Can you work these out from the drawing? Everything is in mm from the part's minimum corner. A direction names the side the tool comes from. Coordinates: 2 decimals unless noted, no trailing zeros. Loops run counter-clockwise (first coordinate to the right, second up) from the corner with the lowest first, then second, coordinate; pieces in that order, holes last. Notation, with made-up numbers: M -16,-13.75 L 1,-13.75 A20 ccw 1,0.25 Z; hole C 3,69 d5. An arc over 180 degrees is marked long. Write each question's results on one line, items separated by ' | '.
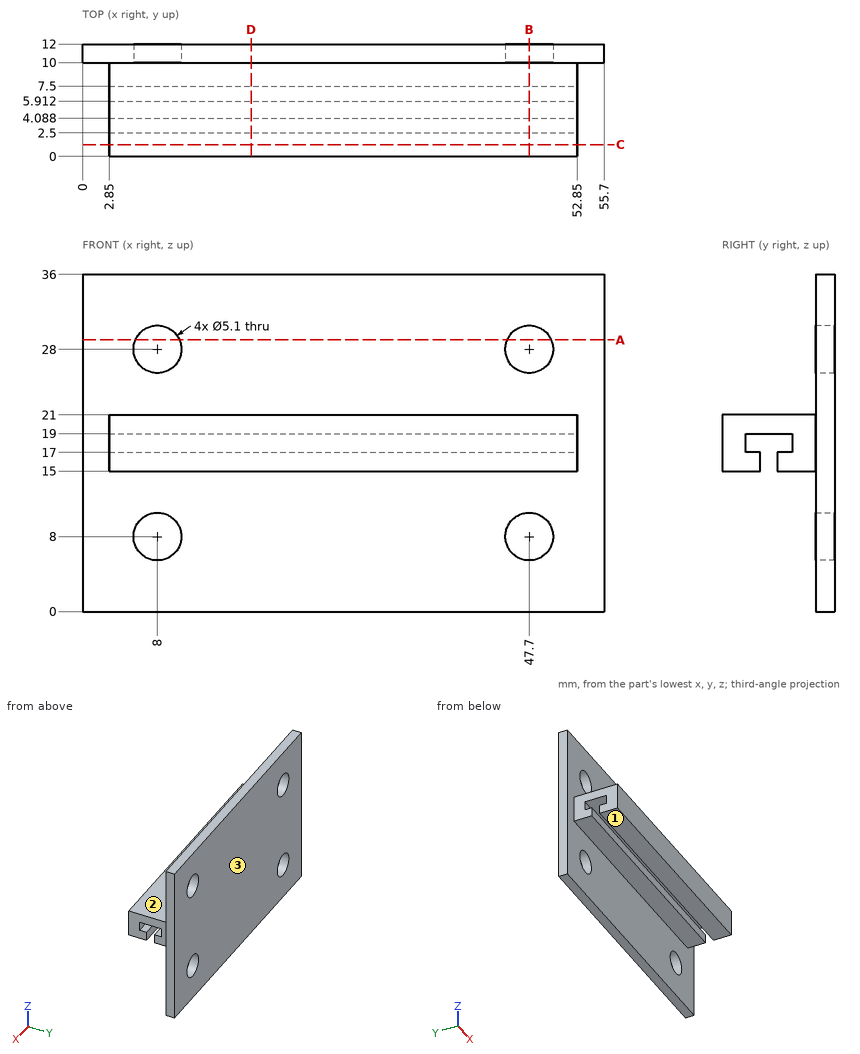
(1) Imagine slicing it at A-A, the plane z = 29. List the corners of the cut face in (x, y) for me (1 decimal).
Reported:
outline: M 0,10 L 5.7,10 L 5.7,12 L 0,12 Z; M 10.3,10 L 45.4,10 L 45.4,12 L 10.3,12 Z; M 50,10 L 55.7,10 L 55.7,12 L 50,12 Z
(2) Which directions (+Z, -Z, +X, -X, +Y, -Y) give clear straight access to the entire face, cutting with the end or side of a thin tool? Please do the marked faces 1, 2 and 3.
Reported:
face 1: -Z, +X, -X, -Y | face 2: +Z, +X, -X, -Y | face 3: +Z, -Z, +X, -X, +Y
(3) Imagine slicing it at B-B, the plane x = 47.7. List the corners of the cut face in (y, z) for me.
Reported:
outline: M 0,15 L 4.09,15 L 4.09,17 L 2.5,17 L 2.5,19 L 7.5,19 L 7.5,17 L 5.91,17 L 5.91,15 L 10,15 L 10,10.55 L 12,10.55 L 12,25.45 L 10,25.45 L 10,21 L 0,21 Z; M 10,0 L 12,0 L 12,5.45 L 10,5.45 Z; M 10,30.55 L 12,30.55 L 12,36 L 10,36 Z
(4) Will these pins go through, and if not, where does the flat tip stop? P1, Ø2, axis at y = 8, z = 19, coming from the -X side; P2, Ø1, axis at x = 29.5, z = 6, coming from the -Y side; P3, Ø1.3, axis at x = 18, y = 3, coming from the +Z side.
Reported:
P1: stops at x = 2.85 | P2: stops at y = 10 | P3: stops at z = 21
(5) Imagine slicing it at C-C, the plane y = 1.25. List the corners of the cut face in (x, z) for me.
Reported:
outline: M 2.85,15 L 52.85,15 L 52.85,21 L 2.85,21 Z
(6) Please list where these lines run through material, in increasing order: probe 1 along X at (y, z) = (10.65, 8); probe 2 along Z at (x, y) = (35, 6); probe 3 along Z at (x, y) = (9, 11.25) (1 decimal). Write a range as from..to.
Reported:
probe 1: x = 0..5.45, 10.55..45.15, 50.25..55.7 | probe 2: z = 15..17, 19..21 | probe 3: z = 0..5.7, 10.3..25.7, 30.3..36
(7) Imagine slicing it at D-D, the plane x = 18. List the corners of the cut face in (y, z) for me, and give its area (3 significant figures).
Reported:
outline: M 0,15 L 4.09,15 L 4.09,17 L 2.5,17 L 2.5,19 L 7.5,19 L 7.5,17 L 5.91,17 L 5.91,15 L 10,15 L 10,0 L 12,0 L 12,36 L 10,36 L 10,21 L 0,21 Z | area: 118 mm2
